Autodesk Inventor part; units mm, degrees
ref_plane "YZ Plane" through (0, 0, 0) normal (1, 0, 0) x (0, 1, 0)
ref_plane "XZ Plane" through (0, 0, 0) normal (0, 1, 0) x (-1, 0, 0)
ref_plane "XY Plane" through (0, 0, 0) normal (0, 0, 1) x (1, 0, 0)
sketch "Sketch1" plane through (0, 0, 0) normal (0, 1, 0) x (-1, 0, 0)
  line L0 (0, 0) -> (190.5, 0)
  line L1 (190.5, 0) -> (47.0141, 19.3142)
  line L2 (47.0141, 19.3142) -> (0, 0)
  line L3 (2.413, -5.8737) -> (-2.413, 5.8737)
  line L4 (-2.413, 5.8737) -> (45.388, 25.5111)
  line L5 (47.0663, 12.4707) -> (2.413, -5.8737)
  line L6 (41.2492, 26.4974) -> (39.555, 13.9109)
  line L7 (48.6964, 12.6805) -> (189.6529, -6.2932)
  line L8 (189.6529, -6.2932) -> (191.3471, 6.2932)
  line L9 (191.3471, 6.2932) -> (47.0181, 25.7209)
  arc A0 (47.0181, 25.7209) -> (45.388, 25.5111) centre (46.5945, 22.5743) ccw
  arc A1 (48.6964, 12.6805) -> (47.0663, 12.4707) centre (48.2728, 9.5338) ccw
  circle A2 centre (47.0141, 19.3142) radius 2.5797
  circle A3 centre (190.5, 0) radius 2.5797
  circle A4 centre (0, 0) radius 2.5797
  line L10 (191.3471, 6.2932) -> (189.6529, -6.2932)
  line L11 (189.6529, -6.2932) -> (192.7995, -6.7168)
  line L12 (196.3697, -3.9937) -> (197.2168, 2.2995)
  line L13 (194.4937, 5.8697) -> (191.3471, 6.2932)
  arc A5 (197.2168, 2.2995) -> (194.4937, 5.8697) centre (194.0702, 2.7231) ccw
  arc A6 (192.7995, -6.7168) -> (196.3697, -3.9937) centre (193.2231, -3.5702) ccw
  line L14 (-2.413, 5.8737) -> (2.413, -5.8737)
  line L15 (2.413, -5.8737) -> (-0.5238, -7.0802)
  line L16 (-4.6672, -5.3498) -> (-7.0802, 0.5238)
  line L17 (-5.3498, 4.6672) -> (-2.413, 5.8737)
  arc A7 (-5.3498, 4.6672) -> (-7.0802, 0.5238) centre (-4.1433, 1.7303) ccw
  arc A8 (-4.6672, -5.3498) -> (-0.5238, -7.0802) centre (-1.7303, -4.1433) ccw
  point P0 (195.9461, -7.1404)
  point P1 (-3.4607, -8.2867)
  dimension "d0" = 190.5
  dimension "d1" = 150
  dimension "d2" = 12.7
  dimension "d3" = 3.175
  dimension "d4" = 5.1594
  dimension "d6" = 6.35
  dimension "d7" = 3.175
  dimension "d8" = 6.35
  dimension "d9" = 3.175
  dimension "d12" = 144.78
extrude "Extrusion1" add sketch "Sketch1" along normal blind 9.525 contours A4 L2 A2 L1 A3 L0 L7 A1 L5 | L0 L5 L3 A4 | A4 L3 L4 L6 L2 | L3 L15 A8 L16 A7 L17 A4 | L6 L4 A0 L9 L8 A3 L1 A2 L2 | L0 A3 L8 L7 | L8 A3 L13 A5 L12 A6 L11
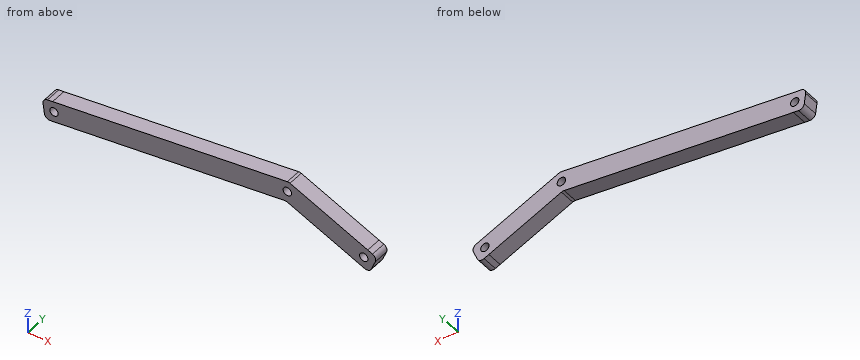
Geometry: final body of the model. Coordinates: model frame, mm. Coordinates: 2 decimals unless noted, no trailing zeros. Order: outer loops, then holes, each group sorted by start corner. A loop starts at its lowest first (then second) coordinate and runs counter-clockwise, first axis right, second up. Notation, with made-up numbers: (66, 43) -> (109, 43) arc R3 ccw to (109, 47) -> close; hole circle Ø10 at (35, 24.25). An arc over 180 degrees is marked (long way). Write item = value, one per line.
(1) Cut plane A-A on z = 9. Return loops of the section in (x, y) (3 decimals), plus the area to 3 significant figures.
Solved:
outline = (-171.238, 0) -> (-76.039, 0) -> (-76.039, 9.525) -> (-171.238, 9.525) -> close; (-38.618, 0) -> (-5.197, 0) -> (-5.197, 9.525) -> (-38.618, 9.525) -> close
area = 1,230 mm²
(2) Cut plane B-B on y = 1.5. Return loops of the section in (x, z).
Solved:
outline = (-197.22, 2.3) -> (-196.37, -3.99) arc R3.17 ccw to (-192.8, -6.72) -> (-189.65, -6.29) -> (-48.7, 12.68) arc R3.17 cw to (-47.07, 12.47) -> (-2.41, -5.87) -> (0.52, -7.08) arc R3.18 ccw to (4.67, -5.35) -> (7.08, 0.52) arc R3.18 ccw to (5.35, 4.67) -> (2.41, 5.87) -> (-45.39, 25.51) arc R3.17 ccw to (-47.02, 25.72) -> (-191.35, 6.29) -> (-194.49, 5.87) arc R3.17 ccw to start; hole circle Ø5.16 at (-190.5, 0); hole circle Ø5.16 at (-47.01, 19.31); hole circle Ø5.16 at (0, 0)
(3) Pin query (flat end, axial travel): pin 1 Ø1 at (x, y) = (-97, 2) entering from -Z; pin 2 Ø4 at (x, y) = (-76.5, 4) entering from +Z; pin 3 Ø1.5 at (x, y) = (-52, 8.5) entering from +Z. Return the tip coordinate at first contact, or that it passes through.
Solved:
pin_1 = 6.11
pin_2 = 22.02
pin_3 = 25.15
(4) Cut plane D-D on x = -29. Return loops of the section in (y, z) (3 decimals), plus the area to 3 significant figures.
Solved:
outline = (0, 5.049) -> (9.525, 5.049) -> (9.525, 18.779) -> (0, 18.779) -> close
area = 131 mm²
(5) Line query: line 1 (Z direction, x = -190.5, y = 5.75); line 2 (Z direction, x = 0, y = 4.75) (3 decimals); line 3 (Z direction, x = -13.5, y = 4). Output: solid intervals per line, ascending.
Solved:
line_1 = -6.41 to -2.58, 2.58 to 6.41
line_2 = -6.865 to -2.58, 2.58 to 6.865
line_3 = -1.32 to 12.41
(6) Cut plane C-C on x = -152. Return loops of the section in (y, z) (3 decimals).
Solved:
outline = (0, -1.225) -> (9.525, -1.225) -> (9.525, 11.59) -> (0, 11.59) -> close
